Could you check a few things on this drawing? It's one solid part, dimensions in mm from its lowest x, y, z. Give positions to 0.01 mm unless a question says otherwise; leave off trailing zeros. Write each loop counter-clockwise with the first axis right and the second up, starting at its lowest first coordinate (ties: lowest second). Pieces come first, ordered by that corner, then holes. Notation, with made-up numbers: (7, -7.5) - (16, -7.5) arc R9 cw to (16, 0.5) - close; hole circle Ø10 at (8.5, 76). An arc over 180 degrees is marked (long way). One line per item, written item: value. Start each with the question number.
1) Imagine slicing it at C-C on y = 8.75. Write out the boundary of the cut face in (x, z) (1 decimal), plus the area to 3 significant figures.
2) Please list where these lines run through material, in increasing order: L1, parallel to Z at x = 13, y = 11.75; L2, parallel to X at y = 12.25, z = 18 (1 decimal); L3, parallel to Z at x = 14.5, y = 4.5 (1 decimal). Write a range as [from, to].
3) Imagine slicing it at D-D on z = 24.5. Write out the boundary of the cut face in (x, y).
4) Imagine slicing it at B-B on z = 15. Write out the boundary of the cut face in (x, y), plus the area to 3 significant figures.
5) We'd pull the mould along X, two halves only. Please class the marked faces 1, 2, 3 and 4: +X half, -X half, draft (parallel to the pull), parting line (faces both ways), or undercut.
6) Imagine slicing it at A-A on x = 14. Write out the boundary of the cut face in (y, z) (1 decimal), plus the area to 3 significant figures.
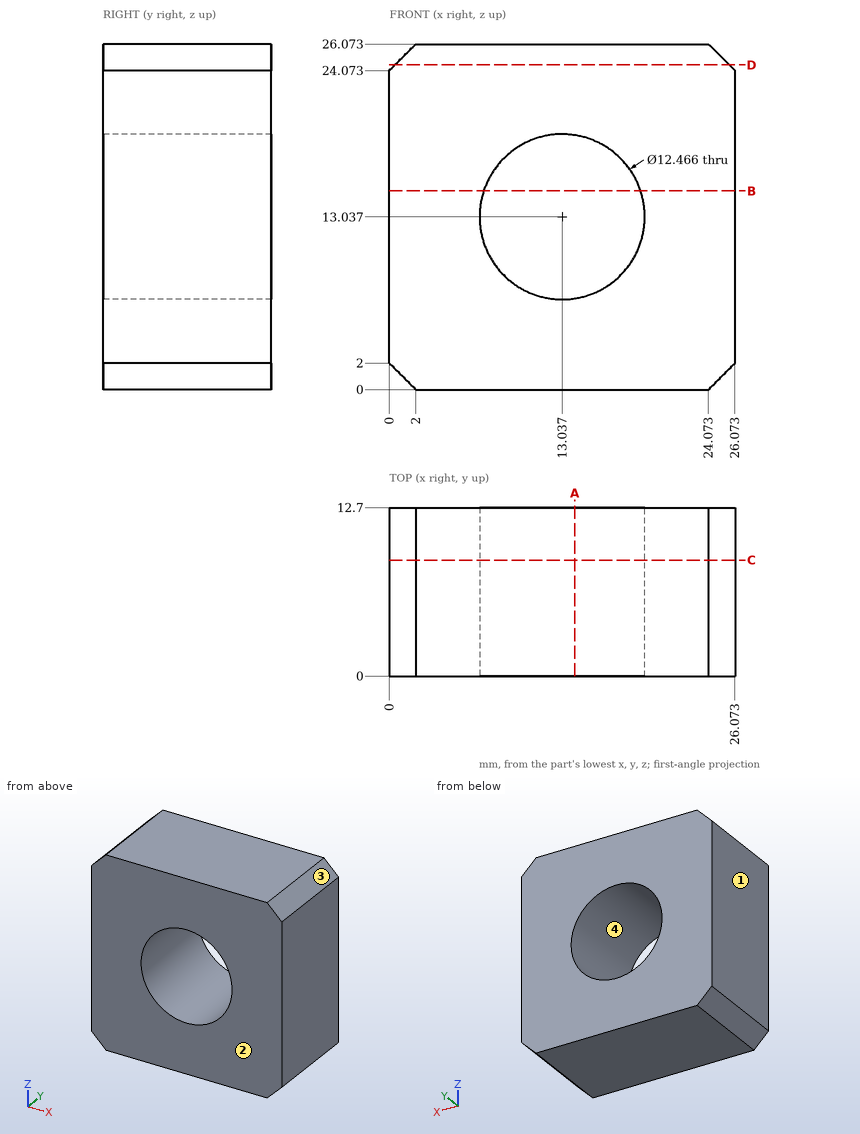
Numbers:
1. outline: (0, 2) - (2, 0) - (24.1, 0) - (26.1, 2) - (26.1, 24.1) - (24.1, 26.1) - (2, 26.1) - (0, 24.1) - close; hole circle Ø12.5 at (13, 13)
1. area: 550 mm^2
2. L1: [0, 6.8], [19.27, 26.07]
2. L2: [0, 9.3], [16.8, 26.1]
2. L3: [0, 7], [19.1, 26.1]
3. outline: (0.43, 0) - (25.65, 0) - (25.65, 12.7) - (0.43, 12.7) - close
4. outline: (0, 0) - (7.12, 0) - (7.12, 12.7) - (0, 12.7) - close; (18.95, 0) - (26.07, 0) - (26.07, 12.7) - (18.95, 12.7) - close
4. area: 181 mm^2
5. face 1: -X half
5. face 2: draft
5. face 3: +X half
5. face 4: undercut
6. outline: (0, 0) - (12.7, 0) - (12.7, 6.9) - (0, 6.9) - close; (0, 19.2) - (12.7, 19.2) - (12.7, 26.1) - (0, 26.1) - close
6. area: 175 mm^2
